Can you work these out from the model? Positions are in its coordinate system, mm. A direction names the side the tool comes from. Coordinates: 2 decimals unless noted, no trailing zeros. Order: outer loops, then holes, each group sorted by start corner. A loop starts at its lowest first (then second) coordinate and runs counter-clockwise, first axis right, second up.
```python
from build123d import *

# Parameters (mm, degrees)
F0_R     = 11.25
F1_DEPTH = 4
F2_R     = 4.5
F3_DEPTH = 6
F6_R     = 2
F7_DEPTH = 4


with BuildPart() as f1:
    # F0 (on Top) → F1 (new body)
    with BuildSketch(Plane.XY):
        Circle(F0_R)
    extrude(amount=F1_DEPTH)

    # F2 (on face) → F3 (join)
    with BuildSketch(Plane.XY.offset(4)):
        Circle(F2_R)
    extrude(amount=F3_DEPTH)

    # F4 (on Front) → F5 (revolve)
    with BuildSketch(Plane.XZ):
        with BuildLine():
            Line((20.5, 15), (0, 15))
            Line((0, 15), (0, 10))
            Line((0, 10), (4.5, 10))
            Line((4.5, 10), (26, 15))
            Line((26, 15), (26, 15.5))
            ThreePointArc((26, 15.5), (25, 16.5), (24, 15.5))
            Line((24, 15.5), (20.5, 15))
        make_face()
    revolve(axis=Axis((0, 0, 19.201497), (0, 0, 1)))

    # F6 (on face) → F7 (cut, through all)
    with BuildSketch(Plane(origin=(0, 0, 0), x_dir=(1, 0, 0), z_dir=(0, 0, -1))):
        with Locations((-5.629165, -3.25)):
            Circle(F6_R)
        with Locations((5.629165, -3.25)):
            Circle(F6_R)
        with Locations((0, 6.5)):
            Circle(F6_R)
    extrude(amount=-F7_DEPTH, mode=Mode.SUBTRACT)


solid = f1.part
```
1. Thinking about a two-plate mould opening in Y: for faces 1 (the flat face through (0, 0, 0)), 2 (the conical face through (2.697, -5.185, 10.313)), 3 (the conical face through (-16.403, -12.577, 15.024)), which applies, pulls with the +Y half, pulls with the -Y half, needs draft (parallel to the pull), parting line crosses it, or undercut?
Completed:
face 1: needs draft
face 2: parting line crosses it
face 3: undercut
2. Imagine slicing it at C-C on z = 2. Please give me the cut outline in (x, y), then the cut area to 3 significant figures.
Completed:
outline: circle Ø22.5 at (0, 0); hole circle Ø4 at (-5.63, 3.25); hole circle Ø4 at (0, -6.5); hole circle Ø4 at (5.63, 3.25)
area: 360 mm2
3. On a 3-axis mill with a long thin cutter (end or side, diameter ignored), from which of +Z, -Z, +X, -X, +Y, -Y can I reach the whole of each face in a straight line? I mean faces 4 (the cylindrical face through (4.042, 4.467, 1.972)), 5 (the flat face through (0, 0, 15)), 6 (the cylindrical face through (-0.59, 4.46, 6.96)). Say none if no direction works.
Completed:
face 4: -Z
face 5: +Z
face 6: none
4. I'm going to push flat-ended pins straight in: pin 1 (4.5 mm diameter, centred on x = -5.63, y = 3.25, fed in from +Z); pin 2 (8 mm diameter, centred on x = 3, z = 11.5, fed in from -Y); pin 3 (1.5 mm diameter, centred on x = -6.5, y = -16.5, fed in from -Z). Where does each tip first touch, or does it pass through?
Completed:
pin 1: stops at z = 15
pin 2: stops at y = -25.98
pin 3: stops at z = 12.9
5. Imagine slicing it at D-D on y = -6.5. Give the number of separate pieces and of enclosed holes in the cut face, then the cut area to 3 significant figures.
Completed:
separate pieces: 3
enclosed holes: 0
area: 197 mm2
6. Imagine slicing it at B-B on z = 8.25. Please give me the cut outline in (x, y), then the cut area to 3 significant figures.
Completed:
outline: circle Ø9 at (0, 0)
area: 63.6 mm2
7. Imagine slicing it at A-A on y = 0. Please give me the cut outline in (x, z).
Completed:
outline: (-26, 15) - (-4.5, 10) - (-4.5, 4) - (-11.25, 4) - (-11.25, 0) - (11.25, 0) - (11.25, 4) - (4.5, 4) - (4.5, 10) - (26, 15) - (26, 15.5) arc R1 ccw to (24, 15.5) - (20.5, 15) - (-20.5, 15) - (-24, 15.5) arc R1 ccw to (-26, 15.5) - close
8. Please list where these lines run through material, in increasing order: probe 1 along X at (y, z) = (3.25, 2.6); probe 2 along X at (y, z) = (-6.5, 1.95); probe 3 along Z at (x, y) = (-10, -4.5).
Completed:
probe 1: x = -10.77 to -7.63, -3.63 to 3.63, 7.63 to 10.77
probe 2: x = -9.18 to -2, 2 to 9.18
probe 3: z = 0 to 4, 11.5 to 15
